Autodesk Inventor part; units mm, degrees
ref_plane "YZ Plane" through (0, 0, 0) normal (1, 0, 0) x (0, 1, 0)
ref_plane "XZ Plane" through (0, 0, 0) normal (0, 1, 0) x (-1, 0, 0)
ref_plane "XY Plane" through (0, 0, 0) normal (0, 0, 1) x (1, 0, 0)
sketch "Sketch1" plane through (0, 0, 0) normal (0, 1, 0) x (-1, 0, 0)
  line L0 (0, 0) -> (50.8, 0)
  line L1 (50.8, 0) -> (50.8, -25.4)
  line L2 (50.8, -25.4) -> (0, -25.4)
  line L3 (0, -25.4) -> (0, 0)
  line L4 (47.625, -22.225) -> (47.625, -3.175)
  line L5 (47.625, -3.175) -> (3.175, -3.175)
  line L6 (3.175, -3.175) -> (3.175, -22.225)
  line L7 (3.175, -22.225) -> (47.625, -22.225)
  dimension "d0" = 50.8
  dimension "d1" = 25.4
  dimension "d2" = 3.175
extrude "Extrusion1" add sketch "Sketch1" along normal blind 886.206
sketch "Sketch2" plane through (-50.8, 0, 0) normal (0, 0, 1) x (1, 0, 0)
  line L0 (50.8, 0) -> (0, 0)
  line L1 (50.8, 0) -> (50.8, 886.206)
  line L2 (0, 886.206) -> (50.8, 886.206)
  line L3 (0, 0) -> (0, 886.206)
  line L4 (0, 0) -> (50.8, 0)
  line L5 (50.8, 0) -> (0, 56.4191)
  line L6 (0, 56.4191) -> (50.8, 56.4191)
  line L7 (50.8, 56.4191) -> (50.8, 0)
  line L8 (50.8, 0) -> (0, 0)
  line L9 (0, 0) -> (0, 56.4191)
  line L10 (0, 56.4191) -> (50.8, 0)
  line L11 (0, 56.4191) -> (21.859, 0)
  line L12 (47.625, 0) -> (3.175, 0)
  dimension "d5" = 48
extrude "Extrusion2" cut sketch "Sketch2" against normal blind 914.4 contours L0 L11 L5 | L11 L0 L3
sketch "Sketch3" plane through (-50.8, 886.206, 0) normal (0, 0, 1) x (1, 0, 0)
  line L0 (0, -829.7869) -> (50.8, -886.206)
  line L1 (50.8, -886.206) -> (50.8, 0)
  line L2 (0, 0) -> (50.8, 0)
  line L3 (0, -829.7869) -> (0, 0)
  line L4 (0, -829.7869) -> (50.8, -886.206)
  line L5 (0, -829.7869) -> (50.8, -784.0464)
  line L6 (50.8, -886.206) -> (50.8, 0)
  line L7 (0, -829.7869) -> (0, 0)
  line L8 (50.8, -886.206) -> (0, -886.206)
  line L9 (0, -886.206) -> (0, -923.3654)
  line L10 (0, -923.3654) -> (50.8, -923.3654)
  line L11 (50.8, -923.3654) -> (50.8, -886.206)
  dimension "d8" = 90
extrude "Extrusion3" cut sketch "Sketch3" against normal blind 25.4 contours L5 L1 L0
sketch "Sketch4" plane through (-50.8, 886.206, 0) normal (0, 0, 1) x (1, 0, 0)
  line L0 (0, -829.7869) -> (50.8, -784.0464)
  line L1 (50.8, -784.0464) -> (50.8, 0)
  line L2 (0, 0) -> (50.8, 0)
  line L3 (0, -829.7869) -> (0, 0)
  line L4 (0, 0) -> (50.8, 0)
  line L5 (0, 0) -> (50.8, 0)
  line L6 (50.8, 0) -> (50.8, -221.7928)
  line L7 (50.8, -221.7928) -> (0, -221.7928)
  line L8 (0, -221.7928) -> (0, 0)
  line L9 (0, -829.7869) -> (0, 0)
  line L10 (0, 0) -> (50.8, -56.4191)
  line L11 (50.8, 0) -> (0, 0)
  line L12 (0, 0) -> (0, -56.4191)
  line L13 (0, -56.4191) -> (50.8, -56.4191)
  line L14 (50.8, -56.4191) -> (50.8, 0)
  point P0 (50.8, -886.206)
  dimension "d11" = 221.7928
  dimension "d12" = 48
  dimension "d13" = 56.4191
extrude "Extrusion4" cut sketch "Sketch4" against normal blind 25.4 contours L10 L2 L1
sketch "Sketch8" plane through (-50.8, 56.4191, 0) normal (0, 0, 1) x (1, 0, 0)
  circle A0 centre (25.4, 702.7869) radius 12.7
  line L0 (0, 0) -> (0, 829.7869)
  circle A1 centre (25.4, 127) radius 12.7
  circle A2 centre (25.4, 406.4) radius 12.7
  point P0 (50.8, -56.4191)
  dimension "d24" = 25.4
  dimension "d25" = 25.4
  dimension "d26" = 127
  dimension "d27" = 25.4
  dimension "d28" = 25.4
  dimension "d29" = 127
  dimension "d32" = 25.4
  dimension "d37" = 279.4
extrude "Extrusion8" cut sketch "Sketch8" against normal blind 25.4
properties part number "AngleBrace.ver1-1111-2020"
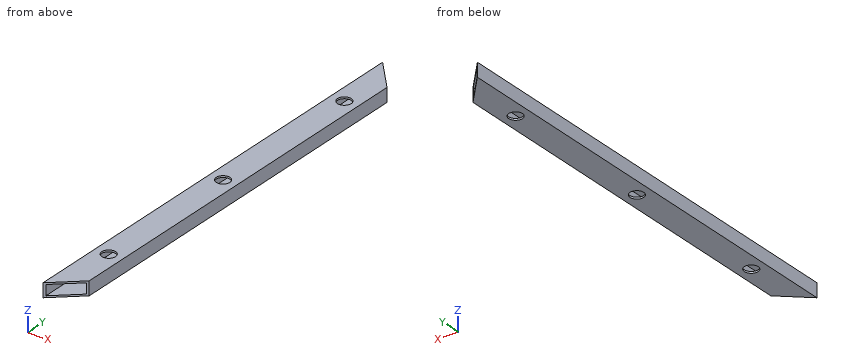
Can you work these out from the model? Positions are in its coordinate system, mm. Round coordinates to 2 decimals unless told otherwise and drop trailing zeros. Order: outer loops, then holes, each group sorted by start corner. A loop starts at its lowest first (then second) coordinate and runs counter-clockwise, first axis right, second up.
(1) If we section it at B-B (x = -22.5): Count the separate pieces of the cut face and the enclosed holes in it, plus the area to 3 significant figures.
Results are:
separate pieces: 8
enclosed holes: 0
area: 4,440 mm2
(2) I'm going to push flat-ended pins straight in: pin 1 (23 mm diameter, centred on x = -25.4, y = 462.82, fed in from -Z); pin 2 (10 mm diameter, centred on x = -8.5, y = 382.5, fed in from +Z). Where does each tip first touch, or does it pass through?
Results are:
pin 1: passes through
pin 2: stops at z = 0
(3) If I drill on L1, parallel to X at y = 182, z = -21 (3 decimals); L2, parallel to Z at x = -36, y = 684.5 (3 decimals); L3, parallel to Y at x = -25.4, z = -23.2, over which ranges is the centre line in solid material (lowest first)?
Results are:
L1: x = -50.8 to -47.625, -3.175 to 0
L2: z = -25.4 to -22.225, -3.175 to 0
L3: y = 79.29 to 170.72, 196.12 to 450.12, 475.52 to 746.51, 771.91 to 858
(4) If we section it at C-C (y = 422): Please give me the cut outline in (x, z) (3 decimals).
Results are:
outline: (-50.8, -25.4) - (0, -25.4) - (0, 0) - (-50.8, 0) - close; hole (-47.625, -22.225) - (-3.175, -22.225) - (-3.175, -3.175) - (-47.625, -3.175) - close
(5) If we section it at A-A (z = -16.75): Please give me the cut outline in (x, y) (3 decimals), plus the area to 3 significant figures.
Results are:
outline: (-50.8, 56.419) - (-47.625, 59.278) - (-47.625, 882.68) - (-50.8, 886.206) - close; (-3.175, 99.301) - (0, 102.16) - (0, 829.787) - (-3.175, 833.313) - close
area: 4,940 mm2
